```python
from build123d import *

# Parameters (mm, degrees)
F2_R     = 0.9271
F3_DEPTH = 12.7
F4_R     = 0.9271
F5_DEPTH = 12.7


with BuildPart() as f1:
    # F0 (on Right) → F1 (revolve)
    with BuildSketch(Plane.YZ):
        Polygon((0, 1.7272), (0, 0), (88.5, 0), (88.5, 1.7272), (67.5, 1.7272), (61.25, 5), (41.25, 5), (35, 1.7272), align=None)
    revolve(axis=Axis((0, 44.25, 0), (0, 1, 0)))

    # F2 (on face) → F3 (cut)
    with BuildSketch(Plane(origin=(0, 88.5, 0), x_dir=(-1, 0, 0), z_dir=(0, 1, 0))):
        Circle(F2_R)
    extrude(amount=-F3_DEPTH, mode=Mode.SUBTRACT)

    # F4 (on face) → F5 (cut)
    with BuildSketch(Plane.XZ):
        Circle(F4_R)
    extrude(amount=-F5_DEPTH, mode=Mode.SUBTRACT)


solid = f1.part
```
Geometry check sheet. Reference: the model listing, model coordinates, mm. A direction names the side the tool comes from. Coordinates: 2 decimals unless noted, no trailing zeros. Write each loop counter-clockwise with the first axis right and the second up, starting at its lowest first coordinate (ties: lowest second). Pieces come first, ordered by that corner, then holes. Notation, with made-up numbers: M 27,72 L 59,72 A10 cw 59,76 Z; hole C 76,81.25 d2. An arc over 180 degrees is marked long. Answer as a JSON object with one key per item and string values.
1. Tool access check on faces 4 (the cylindrical face through (1.713, 77.853, -0.225)), 5 (the flat face through (0, 12.7, 0)), 6 (the flat face through (-1, 88.5, -1)). Record the directions out of +Z, -Z, +X, -X, +Y, -Y that give a thin tool (end or side, any length) a straight path to the whole face; none if there is none.
Answers below:
{"face 4": "+Y", "face 5": "-Y", "face 6": "+Z, -Z, +X, -X, +Y"}
2. Scan lines: L1, parallel to Z at x = 0.25, y = 32; L2, parallel to Z at x = 2.25, y = 40.5; L3, parallel to Y at x = -0.25, z = -3. Record each from-to range of solid material in increasing order.
Answers below:
{"L1": "z = -1.71 to 1.71", "L2": "z = -4.02 to 4.02", "L3": "y = 37.45 to 65.05"}
3. Section check A-A, the plane z = 0. Enter the section's corners in (x, y), plus the area to 3 significant figures.
Answers below:
{"outline": "M -5,41.25 L -1.73,35 L -1.73,0 L -0.93,0 L -0.93,12.7 L 0.93,12.7 L 0.93,0 L 1.73,0 L 1.73,35 L 5,41.25 L 5,61.25 L 1.73,67.5 L 1.73,88.5 L 0.93,88.5 L 0.93,75.8 L -0.93,75.8 L -0.93,88.5 L -1.73,88.5 L -1.73,67.5 L -5,61.25 Z", "area": "430 mm²"}
4. Go/stop test with flat-tipped pins: pin 1 Ø1.1 at (x, z) = (0, 0) entering from -Y; pin 2 Ø6 at (y, z) = (68.5, -3) entering from +X; pin 3 Ø6 at (x, y) = (3.5, 13.5) entering from -Z. Record where each tip stops, or that it passes through.
Answers below:
{"pin 1": "stops at y = 12.7", "pin 2": "stops at x = 2.16", "pin 3": "stops at z = -1.65"}
5. Draft check along Z on faces 1 (the cylindrical face through (0.43, 6.26, -0.82)), 2 (the flat face through (-1, 0, 1)), 3 (the cylindrical face through (1.713, 17.255, -0.225)). Enter one of: released by +Z, released by -Z, zero draft, split by the parting line, or undercut.
Answers below:
{"face 1": "undercut", "face 2": "zero draft", "face 3": "split by the parting line"}
6. Section check D-D, the plane y = 19.5. Enter the section's corners in (x, z).
Answers below:
{"outline": "C 0,0 d3.45"}
7. Section check B-B, the plane x = 0. Enter the section's corners in (y, z).
Answers below:
{"outline": "M 0,-1.73 L 35,-1.73 L 41.25,-5 L 61.25,-5 L 67.5,-1.73 L 88.5,-1.73 L 88.5,-0.93 L 75.8,-0.93 L 75.8,0.93 L 88.5,0.93 L 88.5,1.73 L 67.5,1.73 L 61.25,5 L 41.25,5 L 35,1.73 L 0,1.73 L 0,0.93 L 12.7,0.93 L 12.7,-0.93 L 0,-0.93 Z"}
8. Section check C-C, the plane y = 9.5. Enter the section's corners in (x, z).
Answers below:
{"outline": "C 0,0 d3.45; hole C 0,0 d1.85"}
